The model under review builds one solid part; all positions refer to its coordinate system, in mm. Face numbers are marked on the shaded views. A direction names the side the tool comes from. Round coordinates to 2 decimals unless told otherwise and drop trailing zeros. Write each loop counter-clockwise with the first axis right and the second up, starting at its lowest first coordinate (ties: lowest second). Pieces come first, ordered by that corner, then holes. Notation, with made-up numbers: (78.5, 52.5) -> (135.5, 52.5) arc R21 cw to (135.5, 68.5) -> close; hole circle Ø3 at (43, 64.25). An arc over 180 degrees is marked (long way). Answer in a Markdown table with one row per item. Add a question column.
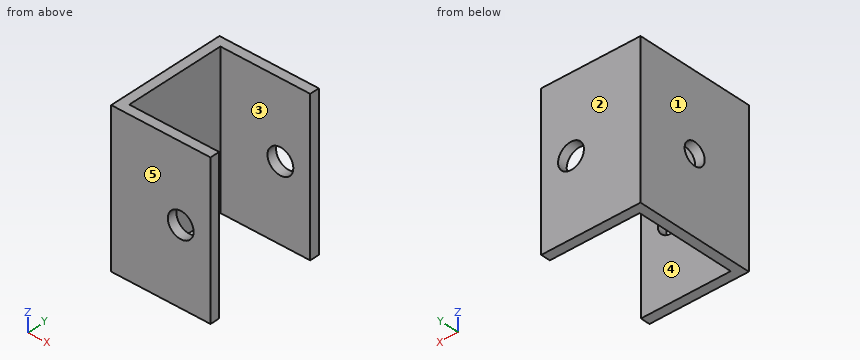
```python
from build123d import *

# Parameters (mm, degrees)
SALIENTE_EXTRUIR3_DEPTH = 38.1
CROQUIS7_R              = 5.55625
CORTAR_EXTRUIR1_DEPTH   = 5
CROQUIS8_R              = 6.5
CORTAR_EXTRUIR2_DEPTH   = 70


with BuildPart() as part:
    # Croquis6 → Saliente-Extruir3 (new, symmetric)
    with BuildSketch(Plane.XY):
        Polygon((45.2375, 25.2375), (0, 25.2375), (0, -25.2375), (45.2375, -25.2375), (45.2375, -30), (-4.7625, -30), (-4.7625, 30), (45.2375, 30), align=None)
    extrude(amount=SALIENTE_EXTRUIR3_DEPTH, both=True)

    # Croquis7 → Cortar-Extruir1 (cut)
    with BuildSketch(Plane.ZY.offset(4.7625)):
        with Locations(Location((0, 0, 0), (0, 0, 270))):
            Circle(CROQUIS7_R)
    extrude(amount=-CORTAR_EXTRUIR1_DEPTH, mode=Mode.SUBTRACT)

    # Croquis8 → Cortar-Extruir2 (cut)
    with BuildSketch(Plane.XZ.offset(30)):
        with Locations((30.2375, 0)):
            Circle(CROQUIS8_R)
    extrude(amount=-CORTAR_EXTRUIR2_DEPTH, mode=Mode.SUBTRACT)


solid = part.part
```
1. Add section A-A on x = 15. Write out the cut boundary in (y, z), plus the area to 3 significant figures.
2. Mouldability with a two-part tool opening along Y and no side actions: class the marked faces 1, 2 and 3 as pulls with the +Y half, pulls with the -Y half, needs draft (parallel to the pull), parting line crosses it, or undercut.
3. Tool access review of the marked faces 4 and 5: name each direction out of +Z, -Z, +X, -X, +Y, -Y from which nothing blocks a thin tool from reaching the whole face with its end or side.
4. Insertion check: pin 1 Ø6.5 at (y, z) = (0, 0) entering from +X; pin 2 Ø25 at (y, z) = (3, 7) entering from +X. Each pin has a flat end and moves straight along its axis. Give the tip position at first contact, or say it passes through.
5. For L1, parallel to Y at x = 26, z = 19; L2, parallel to Y at x = -2, z = 0.5; L3, parallel to X at y = 0.5, z = 28, list the stretches that pass through material, from the lowest coordinate up.
6. Add section C-C on y = 0. Write out the cut boundary in (x, z), plus the area to 3 significant figures.
7. Add section B-B on z = 0. Write out the cut boundary in (x, y), plus the area to 3 significant figures.
8. Add section D-D on x = 31. Write out the cut boundary in (y, z), plus the area to 3 significant figures.
Filled in:
| question | item | result |
|---|---|---|
| 1 | outline | (-30, -38.1) -> (-25.24, -38.1) -> (-25.24, 38.1) -> (-30, 38.1) -> close; (25.24, -38.1) -> (30, -38.1) -> (30, 38.1) -> (25.24, 38.1) -> close |
| 1 | area | 726 mm² |
| 2 | face 1 | needs draft |
| 2 | face 2 | pulls with the +Y half |
| 2 | face 3 | undercut |
| 3 | face 4 | +Z, -Z, +X |
| 3 | face 5 | +Z, -Z, +X, -X, -Y |
| 4 | pin 1 | through |
| 4 | pin 2 | x = 0 |
| 5 | L1 | -30 to -25.24, 25.24 to 30 |
| 5 | L2 | -30 to -5.53, 5.53 to 30 |
| 5 | L3 | -4.76 to 0 |
| 6 | outline | (-4.76, -38.1) -> (0, -38.1) -> (0, -5.56) -> (-4.76, -5.56) -> close; (-4.76, 5.56) -> (0, 5.56) -> (0, 38.1) -> (-4.76, 38.1) -> close |
| 6 | area | 310 mm² |
| 7 | outline | (-4.76, -30) -> (23.74, -30) -> (23.74, -25.24) -> (0, -25.24) -> (0, -5.56) -> (-4.76, -5.56) -> close; (-4.76, 5.56) -> (0, 5.56) -> (0, 25.24) -> (23.74, 25.24) -> (23.74, 30) -> (-4.76, 30) -> close; (36.74, -30) -> (45.24, -30) -> (45.24, -25.24) -> (36.74, -25.24) -> close; (36.74, 25.24) -> (45.24, 25.24) -> (45.24, 30) -> (36.74, 30) -> close |
| 7 | area | 540 mm² |
| 8 | outline | (-30, -38.1) -> (-25.24, -38.1) -> (-25.24, -6.46) -> (-30, -6.46) -> close; (-30, 6.46) -> (-25.24, 6.46) -> (-25.24, 38.1) -> (-30, 38.1) -> close; (25.24, -38.1) -> (30, -38.1) -> (30, -6.46) -> (25.24, -6.46) -> close; (25.24, 6.46) -> (30, 6.46) -> (30, 38.1) -> (25.24, 38.1) -> close |
| 8 | area | 603 mm² |
